Read the model definition and answer for the solid it produces. Units are mm, in the model's axes. Face numbers are marked on the shaded views. A direction names the side the tool comes from. Give positions to 0.01 mm unless a question says otherwise; leave off trailing zeros. Order: outer loops, then holes, each group sorted by start corner. A loop starts at its lowest first (then second) coordinate and runs counter-clockwise, first axis right, second up. Notation, with made-up numbers: (50, 40) - (56, 40) arc R21 cw to (56, 45) - close; hole circle Ø10 at (-36.5, 87). An arc over 180 degrees is marked (long way). Return JSON: item names as keys, results as strings.
```python
from build123d import *

# Parameters (mm, degrees)
F1_DEPTH = 2.36
F0_W     = 14
F0_H     = 5.7202167809
F0_R     = 2.25
F0_R_2   = 4.5
F2_DEPTH = 0.5
F3_R     = 0.49999
F4_DEPTH = 1.36
F5_DEPTH = 1.36


# Not quite as in the source:
# - a fillet or chamfer is up to 0.001 mm smaller than in the source, because OpenCascade refuses the exact size


with BuildPart() as f1:
    # F0 (on Top) → F1 (new body)
    with BuildSketch(Plane.XY):
        with BuildLine():
            ThreePointArc((-2, -1), (-1.7071067812, -1.7071067812), (-1, -2))
            Line((-1, -2), (15, -2))
            ThreePointArc((15, -2), (15.7071067812, -1.7071067812), (16, -1))
            Line((16, -1), (16, 30))
            ThreePointArc((16, 30), (15.7071067812, 30.7071067812), (15, 31))
            Line((15, 31), (13, 31))
            Line((13, 31), (13, 42))
            ThreePointArc((13, 42), (12.7071067812, 42.7071067812), (12, 43))
            Line((12, 43), (2, 43))
            ThreePointArc((2, 43), (1.2928932188, 42.7071067812), (1, 42))
            Line((1, 42), (1, 31))
            Line((1, 31), (-1, 31))
            ThreePointArc((-1, 31), (-1.7071067812, 30.7071067812), (-2, 30))
            Line((-2, 30), (-2, -1))
        make_face()
        Polygon((14, 0), (0, 0), (0, 5.7202167809), (0, 29), (2.5, 29), (2.5, 31), (2.5, 42), (4.75, 42), (4.75, 41), (9.25, 41), (9.25, 42), (11.5, 42), (11.5, 31), (11.5, 29), (14, 29), (14, 5.7202167809), align=None, mode=Mode.SUBTRACT)
    extrude(amount=F1_DEPTH)

    # F0 (on Top) → F2 (join)
    with BuildSketch(Plane.XY):
        with BuildLine():
            ThreePointArc((-2, -1), (-1.7071067812, -1.7071067812), (-1, -2))
            Line((-1, -2), (15, -2))
            ThreePointArc((15, -2), (15.7071067812, -1.7071067812), (16, -1))
            Line((16, -1), (16, 30))
            ThreePointArc((16, 30), (15.7071067812, 30.7071067812), (15, 31))
            Line((15, 31), (13, 31))
            Line((13, 31), (13, 42))
            ThreePointArc((13, 42), (12.7071067812, 42.7071067812), (12, 43))
            Line((12, 43), (2, 43))
            ThreePointArc((2, 43), (1.2928932188, 42.7071067812), (1, 42))
            Line((1, 42), (1, 31))
            Line((1, 31), (-1, 31))
            ThreePointArc((-1, 31), (-1.7071067812, 30.7071067812), (-2, 30))
            Line((-2, 30), (-2, -1))
        make_face()
        Polygon((14, 0), (0, 0), (0, 5.7202167809), (0, 29), (2.5, 29), (2.5, 31), (2.5, 42), (4.75, 42), (4.75, 41), (9.25, 41), (9.25, 42), (11.5, 42), (11.5, 31), (11.5, 29), (14, 29), (14, 5.7202167809), align=None, mode=Mode.SUBTRACT)
        with Locations((7, 2.8601083905)):
            Rectangle(F0_W, F0_H)
        with Locations((7, 2.95)):
            Circle(F0_R, mode=Mode.SUBTRACT)
        Polygon((2.5, 42), (2.5, 31), (11.5, 31), (11.5, 42), (9.25, 42), (9.25, 41), (4.75, 41), (4.75, 42), align=None)
        Polygon((0, 29), (0, 5.7202167809), (14, 5.7202167809), (14, 29), (11.5, 29), (11.5, 31), (2.5, 31), (2.5, 29), align=None)
        with Locations((7, 18.8)):
            Circle(F0_R_2, mode=Mode.SUBTRACT)
        with Locations((7, 18.8)):
            Circle(F0_R_2)
    extrude(amount=-F2_DEPTH)

    # F3 (radius 0.5 in the source; OpenCascade refuses exactly that, so slightly less here)
    f3_edges = [f1.edges().sort_by_distance(p)[0] for p in [
        (1, 36.5, -0.5),
        (0, 31, -0.5),
        (-1.707107, 30.707107, -0.5),
        (-2, 14.5, -0.5),
        (-1.707107, -1.707107, -0.5),
        (7, -2, -0.5),
        (15.707107, -1.707107, -0.5),
        (16, 14.5, -0.5),
        (15.707107, 30.707107, -0.5),
        (14, 31, -0.5),
        (13, 36.5, -0.5),
        (12.707107, 42.707107, -0.5),
        (7, 43, -0.5),
        (1.292893, 42.707107, -0.5),
        (4.75, 2.95, -0.5),
    ]]
    fillet(f3_edges, radius=F3_R)

    # F0 (on Top) → F4 (join)
    with BuildSketch(Plane.XY):
        Polygon((2.5, 42), (2.5, 31), (11.5, 31), (11.5, 42), (9.25, 42), (9.25, 41), (4.75, 41), (4.75, 42), align=None)
    extrude(amount=F4_DEPTH)

    # F0 (on Top) → F5 (join)
    with BuildSketch(Plane.XY):
        with Locations((7, 2.8601083905)):
            Rectangle(F0_W, F0_H)
        with Locations((7, 2.95)):
            Circle(F0_R, mode=Mode.SUBTRACT)
    extrude(amount=F5_DEPTH)


solid = f1.part
```
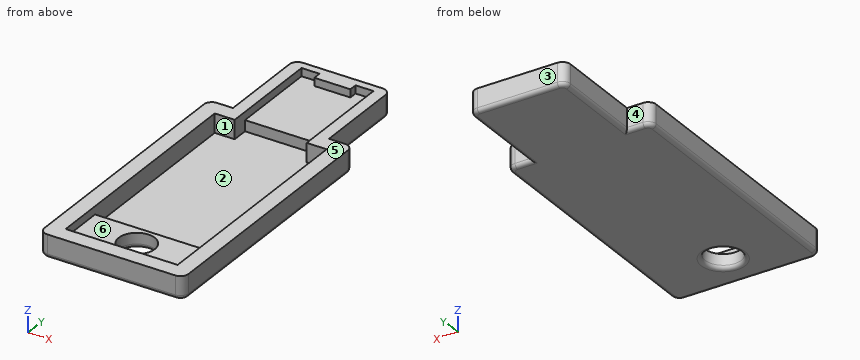
Q1. Consider L1, parallel to Y at x = 7, z = 0.9; L2, parallel to X at y = 37, z = 2.2; L3, parallel to Y at x = 10, z = 0.6. Determine where each line is inside the solid, lowest interval first.
Values:
{"L1": "y = -2 to 0.7, 5.2 to 5.72, 31 to 43", "L2": "x = 1 to 2.5, 11.5 to 13", "L3": "y = -2 to 5.72, 31 to 43"}
Q2. A cutting plane is placed at C-C (z = 1.85). Write down the section's boundary in (x, y).
Values:
{"outline": "(-2, -1) arc R1 ccw to (-1, -2) - (15, -2) arc R1 ccw to (16, -1) - (16, 30) arc R1 ccw to (15, 31) - (13, 31) - (13, 42) arc R1 ccw to (12, 43) - (2, 43) arc R1 ccw to (1, 42) - (1, 31) - (-1, 31) arc R1 ccw to (-2, 30) - close; hole (0, 0) - (14, 0) - (14, 29) - (11.5, 29) - (11.5, 42) - (9.25, 42) - (9.25, 41) - (4.75, 41) - (4.75, 42) - (2.5, 42) - (2.5, 29) - (0, 29) - close"}
Q3. Determine the mould class of the marked faces 1, 2 and 3 for opening direction X: released by +X, released by -X, zero draft, split by the parting line, or undercut.
Values:
{"face 1": "undercut", "face 2": "undercut", "face 3": "zero draft"}
Q4. For the marked faces 4, 5 and 6, determine the directions among +Z, -Z, +X, -X, +Y, -Y from which every point of the face is accessible in a straight line to the end or side of a thin tool.
Values:
{"face 4": "+Z, -Z, -X, +Y", "face 5": "+Z, +X, -X, +Y, -Y", "face 6": "+Z"}
Q5. A cutting plane is placed at B-B (x = 7). Write down the section's boundary in (y, z), and give its area (3 significant figures).
Values:
{"outline": "(-2, 0) arc R0.5 ccw to (-1.5, -0.5) - (0.2, -0.5) arc R0.5 ccw to (0.7, 0) - (0.7, 1.36) - (0, 1.36) - (0, 2.36) - (-2, 2.36) - close; (5.2, 0) arc R0.5 ccw to (5.7, -0.5) - (42.5, -0.5) arc R0.5 ccw to (43, 0) - (43, 2.36) - (41, 2.36) - (41, 1.36) - (31, 1.36) - (31, 0) - (5.72, 0) - (5.72, 1.36) - (5.2, 1.36) - close", "area": "44.7 mm²"}
Q6. Given pin 1 (0.7 mm diameter, centred on y = 34, z = 1.5, fed in from -X); pin 2 (4.5 mm diameter, centred on x = 6.5, y = 35.5, fed in from +Z); pin 3 (0.7 mm diameter, centred on y = 35.5, z = 1, fed in from +X), each flat-ended and moving along its own axis, determine where each tip first touches the part or whether it passes through.
Values:
{"pin 1": "stops at x = 1", "pin 2": "stops at z = 1.36", "pin 3": "stops at x = 13"}
Q7. A cutting plane is placed at D-D (y = 36.5). Write down the section's boundary in (x, z), and give its area (3 significant figures).
Values:
{"outline": "(1, 0) arc R0.5 ccw to (1.5, -0.5) - (12.5, -0.5) arc R0.5 ccw to (13, 0) - (13, 2.36) - (11.5, 2.36) - (11.5, 1.36) - (2.5, 1.36) - (2.5, 2.36) - (1, 2.36) - close", "area": "25.2 mm²"}
Q8. A cutting plane is placed at A-A (y = 2.95). Write down the section's boundary in (x, z), and give its area (3 significant figures).
Values:
{"outline": "(-2, 0) arc R0.5 ccw to (-1.5, -0.5) - (4.25, -0.5) arc R0.5 ccw to (4.75, 0) - (4.75, 1.36) - (0, 1.36) - (0, 2.36) - (-2, 2.36) - close; (9.25, 0) arc R0.5 ccw to (9.75, -0.5) - (15.5, -0.5) arc R0.5 ccw to (16, 0) - (16, 2.36) - (14, 2.36) - (14, 1.36) - (9.25, 1.36) - close", "area": "28.9 mm²"}
